Geometry check sheet. Reference: drawing and pictorial views, mm from the part's lowest x, y, z. Coordinates: 2 decimals unless noted, no trailing zeros. Write each loop counter-clockwise with the first axis right and the second up, starting at its lowest first coordinate (ties: lowest second). Pieces come first, ordered by that corner, then holes. Notation, with made-up numbers: (47, 55.5) -> (88, 55.5) arc R31 ccw to (88, 88.5) -> close; hole circle Ø9 at (80, 17). An arc over 180 degrees is marked (long way). Use a Markdown table: item, result.
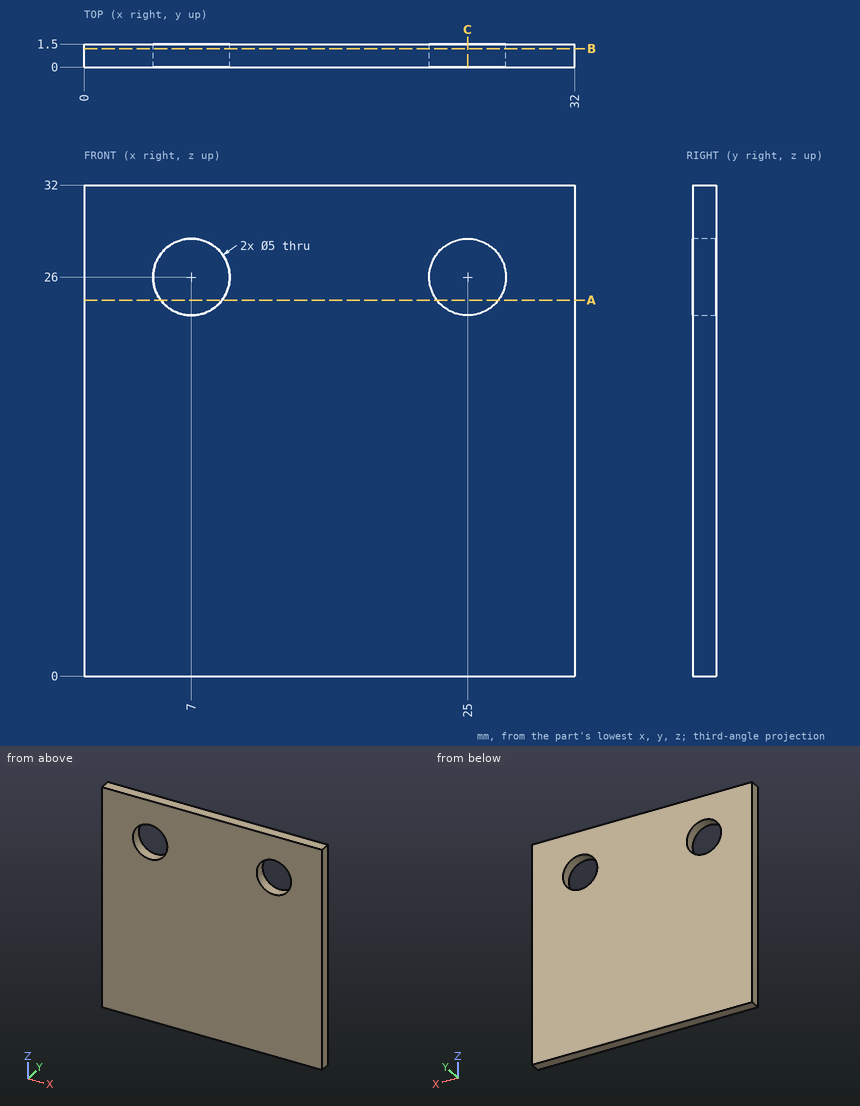
Item 1: Section check B-B on y = 1.2. Record the boundary of the cut face in (x, z).
Answer block:
| item | result |
|---|---|
| outline | (0, 0) -> (32, 0) -> (32, 32) -> (0, 32) -> close; hole circle Ø5 at (7, 26); hole circle Ø5 at (25, 26) |
Item 2: Thickness scan on L1, parallel to X at y = 0.3, z = 26; L2, parallel to Z at x = 7, y = 1.2; L3, parallel to Z at x = 5.5, y = 0.6. Record the ranges inside material, lowest first. Write a range as [from, to].
Answer block:
| item | result |
|---|---|
| L1 | x = [0, 4.5], [9.5, 22.5], [27.5, 32] |
| L2 | z = [0, 23.5], [28.5, 32] |
| L3 | z = [0, 24], [28, 32] |
Item 3: Section check C-C on x = 25. Record the boundary of the cut face in (y, z), then the cut area to 3 significant figures.
Answer block:
| item | result |
|---|---|
| outline | (0, 0) -> (1.5, 0) -> (1.5, 23.5) -> (0, 23.5) -> close; (0, 28.5) -> (1.5, 28.5) -> (1.5, 32) -> (0, 32) -> close |
| area | 40.5 mm^2 |
Item 4: Section check A-A on z = 24.5. Record the boundary of the cut face in (x, y), then the cut area to 3 significant figures.
Answer block:
| item | result |
|---|---|
| outline | (0, 0) -> (5, 0) -> (5, 1.5) -> (0, 1.5) -> close; (9, 0) -> (23, 0) -> (23, 1.5) -> (9, 1.5) -> close; (27, 0) -> (32, 0) -> (32, 1.5) -> (27, 1.5) -> close |
| area | 36.0 mm^2 |
